Geometry: see drawing. Coordinates: mm, zero at the bounding-box minimum. Give positions to 0.01 mm unless a question says otherwise; leave off trailing zeros. Order: outer loops, then holes, each group sorted by start corner. A loop starts at its lowest first (then second) coordinate and runs counter-clockwise, first axis right, second up. Notation, with made-up numbers: (20, -3) -> (57, -3) arc R34 cw to (57, 32) -> close; hole circle Ø1 at (89.5, 79). An arc over 180 degrees is marked (long way). Use one line per item in the form item = value. Start each with the question number.
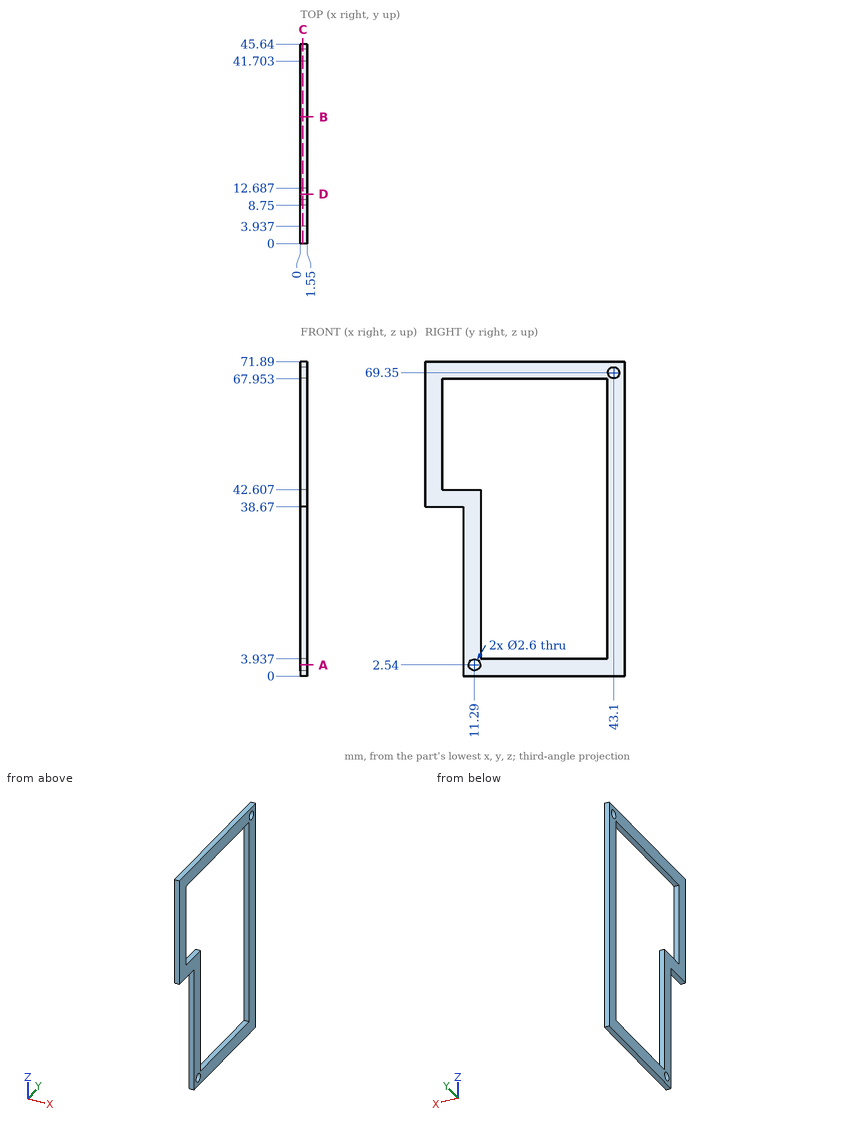
1) Cut plane C-C, the plane x = 0.6. Return the cut outline in (y, z), plus the area to 3 significant figures.
2) Pin query (flat end, axial travel): pin 1 (0.8 mm diameter, centred on x = 1, z = 18, fed in from -Y). Return the tip coordinate at first contact, or that it passes through.
3) Cut plane D-D, the plane y = 11.29. Return the cut outline in (x, z).
4) Cut plane B-B, the plane y = 29. Return the cut outline in (x, z), plus the area to 3 significant figures.
5) Cut plane A-A, the plane z = 2.54. Return the cut outline in (x, y), plus the area to 3 significant figures.
6) Material intervals for probe 1 along Y at (x, z) = (0.75, 2.54); probe 2 along Z at (x, y) = (0.1, 7); probe 3 along Z at (x, y) = (1.1, 43.1), sorted ascending.
Output values:
q1.outline = (0, 38.67) -> (8.75, 38.67) -> (8.75, 0) -> (45.64, 0) -> (45.64, 71.89) -> (0, 71.89) -> close; hole (3.94, 42.61) -> (12.69, 42.61) -> (12.69, 3.94) -> (41.7, 3.94) -> (41.7, 67.95) -> (3.94, 67.95) -> close; hole circle Ø2.6 at (11.29, 2.54); hole circle Ø2.6 at (43.1, 69.35)
q1.area = 853 mm^2
q2.pin_1 = 8.75
q3.outline = (0, 0) -> (1.55, 0) -> (1.55, 1.24) -> (0, 1.24) -> close; (0, 3.84) -> (1.55, 3.84) -> (1.55, 42.61) -> (0, 42.61) -> close; (0, 67.95) -> (1.55, 67.95) -> (1.55, 71.89) -> (0, 71.89) -> close
q4.outline = (0, 0) -> (1.55, 0) -> (1.55, 3.94) -> (0, 3.94) -> close; (0, 67.95) -> (1.55, 67.95) -> (1.55, 71.89) -> (0, 71.89) -> close
q4.area = 12.2 mm^2
q5.outline = (0, 8.75) -> (1.55, 8.75) -> (1.55, 9.99) -> (0, 9.99) -> close; (0, 12.59) -> (1.55, 12.59) -> (1.55, 45.64) -> (0, 45.64) -> close
q5.area = 53.1 mm^2
q6.probe_1 = 8.75 to 9.99, 12.59 to 45.64
q6.probe_2 = 38.67 to 42.61, 67.95 to 71.89
q6.probe_3 = 0 to 68.05, 70.65 to 71.89
